Here's how the part is built. I have some questions about the finished solid (model axes, mm). Round coordinates to 2 decimals unless told otherwise and drop trailing zeros. Loops run counter-clockwise (first coordinate to the right, second up) from the corner with the lowest first, then second, coordinate; pieces in that order, holes last. Notation, with made-up numbers: (28.25, 26) -> (64.25, 26) arc R32 ccw to (64.25, 63) -> close; hole circle Ø1 at (42, 44). An arc over 180 degrees is marked (long way). Use one line per item in the form item = value. Start each with the question number.
Item 1: If I drill on L1, parallel to Z at x = 144.78, y = 0.75; L2, parallel to Z at x = 98, y = 1.15; L3, parallel to X at y = 0.15, z = 95, over which ranges is the centre line in solid material (lowest first)? Write a range as [from, to].
Item 2: If we section it at D-D (y = 1.2): State how many separate pieces and enclosed holes the cut face has, then the cut area to 3 significant figures.
Item 3: If we section it at C-C (x = 109.22): Write out the boundary of the cut face in (y, z).
Item 4: If we section it at A-A (x = 191.38): Write out the boundary of the cut face in (y, z), then the cut area to 3 significant figures.
Item 5: If we section it at B-B (z = 63.08): Write out the boundary of the cut face in (x, y).
Item 6: Thinking about a two-plate mould opening in X: for faces 1 (the face through (125, 1.5, 48)), 2 (the face through (25.91, 0.74, 96.75)), 3 (the face through (180, 1, 5)), which applies, released by +X, released by -X, zero draft, split by the parting line, or undercut?
Item 7: I'm going to push a flat-ended pin straight in: pin 1 Ø0.8 at (x, y) = (131, 0.5) entering from +Z. Where does the tip first touch, or does it pass through?
```python
from build123d import *

# Parameters (mm, degrees)
SKETCH1_R           = 2.3
BOSS_EXTRUDE1_DEPTH = 1.5


with BuildPart() as part:
    # Sketch1 → Boss-Extrude1 (new body)
    with BuildSketch(Plane(origin=(0, 0, 0), x_dir=(1, 0, 0), z_dir=(0, 1, 0))):
        Polygon((52.556347973, -126.995854643), (114.3, -126.995854643), (114.3, -50.8), (139.7, -50.8), (139.7, -126.995854643), (201.436197447, -126.995854643), (254, -67.34), (254, 0), (0, 0), (0, -67.34), align=None)
        with Locations(Location((5.08, -5.08, 0), (0, 0, 270))):
            Circle(SKETCH1_R, mode=Mode.SUBTRACT)
        with Locations(Location((53.03, -5.08, 0), (0, 0, 270))):
            Circle(SKETCH1_R, mode=Mode.SUBTRACT)
        with Locations(Location((99.06, -5.08, 0), (0, 0, 270))):
            Circle(SKETCH1_R, mode=Mode.SUBTRACT)
        with Locations(Location((5.08, -63.08, 0), (0, 0, 270))):
            Circle(SKETCH1_R, mode=Mode.SUBTRACT)
        with Locations(Location((99.066197447, -121.915854643, 0), (0, 0, 270))):
            Circle(SKETCH1_R, mode=Mode.SUBTRACT)
        with Locations(Location((55.856197447, -121.915854643, 0), (0, 0, 270))):
            Circle(SKETCH1_R, mode=Mode.SUBTRACT)
        with Locations(Location((182.3, -5.08, 0), (0, 0, 270))):
            Circle(SKETCH1_R, mode=Mode.SUBTRACT)
        with Locations(Location((248.919999642, -5.086414302, 0), (0, 0, 270))):
            Circle(SKETCH1_R, mode=Mode.SUBTRACT)
        with Locations(Location((248.92, -63.086414302, 0), (0, 0, 270))):
            Circle(SKETCH1_R, mode=Mode.SUBTRACT)
        with Locations(Location((198.136197447, -121.915854643, 0), (0, 0, 270))):
            Circle(SKETCH1_R, mode=Mode.SUBTRACT)
        with Locations(Location((154.926197447, -121.915854643, 0), (0, 0, 270))):
            Circle(SKETCH1_R, mode=Mode.SUBTRACT)
        with Locations(Location((144.78, -5.08, 0), (0, 0, 270))):
            Circle(SKETCH1_R, mode=Mode.SUBTRACT)
        with Locations(Location((109.22, -5.08, 0), (0, 0, 270))):
            Circle(SKETCH1_R, mode=Mode.SUBTRACT)
        with Locations(Location((154.94, -5.08, 0), (0, 0, 270))):
            Circle(SKETCH1_R, mode=Mode.SUBTRACT)
        with Locations(Location((191.38, -5.08, 0), (0, 0, 270))):
            Circle(SKETCH1_R, mode=Mode.SUBTRACT)
        with Locations(Location((223.528114705, -94.239074881, 0), (0, 0, 270))):
            Circle(SKETCH1_R, mode=Mode.SUBTRACT)
        with Locations(Location((144.78, -98.385854643, 0), (0, 0, 270))):
            Circle(SKETCH1_R, mode=Mode.SUBTRACT)
        with Locations(Location((144.78, -83.815854643, 0), (0, 0, 270))):
            Circle(SKETCH1_R, mode=Mode.SUBTRACT)
        with Locations(Location((144.78, -69.245854643, 0), (0, 0, 270))):
            Circle(SKETCH1_R, mode=Mode.SUBTRACT)
        with Locations(Location((109.22, -70.245854643, 0), (0, 0, 270))):
            Circle(SKETCH1_R, mode=Mode.SUBTRACT)
        with Locations(Location((109.22, -84.815854643, 0), (0, 0, 270))):
            Circle(SKETCH1_R, mode=Mode.SUBTRACT)
        with Locations(Location((109.22, -99.385854643, 0), (0, 0, 270))):
            Circle(SKETCH1_R, mode=Mode.SUBTRACT)
        with Locations(Location((30.466395088, -94.237134728, 0), (0, 0, 270))):
            Circle(SKETCH1_R, mode=Mode.SUBTRACT)
    extrude(amount=BOSS_EXTRUDE1_DEPTH)


solid = part.part
```
Values found:
q1.L1 = [0, 2.78], [7.38, 66.95], [71.55, 81.52], [86.12, 96.09], [100.69, 127]
q1.L2 = [0, 3.04], [7.12, 119.88], [123.95, 127]
q1.L3 = [24.37, 28.3], [32.64, 114.3], [139.7, 221.36], [225.7, 229.63]
q2.separate_pieces = 1
q2.enclosed_holes = 23
q2.area = 26,800 mm2
q3.outline = (0, 0) -> (1.5, 0) -> (1.5, 2.78) -> (0, 2.78) -> close; (0, 7.38) -> (1.5, 7.38) -> (1.5, 67.95) -> (0, 67.95) -> close; (0, 72.55) -> (1.5, 72.55) -> (1.5, 82.52) -> (0, 82.52) -> close; (0, 87.12) -> (1.5, 87.12) -> (1.5, 97.09) -> (0, 97.09) -> close; (0, 101.69) -> (1.5, 101.69) -> (1.5, 127) -> (0, 127) -> close
q4.outline = (0, 0) -> (1.5, 0) -> (1.5, 2.78) -> (0, 2.78) -> close; (0, 7.38) -> (1.5, 7.38) -> (1.5, 127) -> (0, 127) -> close
q4.area = 184 mm2
q5.outline = (0, 0) -> (2.78, 0) -> (2.78, 1.5) -> (0, 1.5) -> close; (7.38, 0) -> (114.3, 0) -> (114.3, 1.5) -> (7.38, 1.5) -> close; (139.7, 0) -> (246.62, 0) -> (246.62, 1.5) -> (139.7, 1.5) -> close; (251.22, 0) -> (254, 0) -> (254, 1.5) -> (251.22, 1.5) -> close
q6.face_1 = zero draft
q6.face_2 = released by -X
q6.face_3 = undercut
q7.pin_1 = 50.8
